CAD build for the part. Positions are in the model's coordinates, mm. Face numbers are marked on the shaded views. A direction names the side the tool comes from. Coordinates: 2 decimals unless noted, no trailing zeros. Loops run counter-clockwise (first coordinate to the right, second up) from the corner with the lowest first, then second, coordinate; pieces in that order, holes last.
1) Saw through at A-A, the plane x = 0. Write the cut outline in (y, z).
2) Saw through at C-C, the plane y = 0. Write the cut outline in (x, z), and give its area (3 significant figures).
3) Pin check, flat tips, straight feed: pin 1 Ø3 at (x, y) = (-18, -100) entering from -Z; pin 2 Ø12 at (x, y) = (2.5, -68.5) entering from -Z; pin 3 Ø4 at (x, y) = (-0.5, -91) entering from -Z; pin 4 Ø12 at (y, z) = (-62.5, -61.5) entering from +X. Stop position of each tip, or through.
4) Saw through at B-B, the plane z = -52.5. Write the cut outline in (x, y).
5) Two-plate mould, pull along Y, no slides. Class the marked faces 5, 6 and 7: +Y half, -Y half, draft (parallel to the pull), parting line (faces both ways), or undercut.
6) Which spindle directions (+Z, -Z, +X, -X, +Y, -Y) get a long thin tool onto all of the face, cutting with end or side? Do the marked faces 1, 2, 3 and 4. Say none if no direction does.
7) Wall check: line 1 along Z through (x, y) = (17.5, 14.5); line 2 along Y through (x, z) = (21.5, -60.5); line 3 along Y through (x, z) = (-19.5, -74.5). Give the ranges that are in metal, low to high.
8) Saw through at D-D, the plane x = -10. Write the cut outline in (y, z), and give its area (3 significant figures).
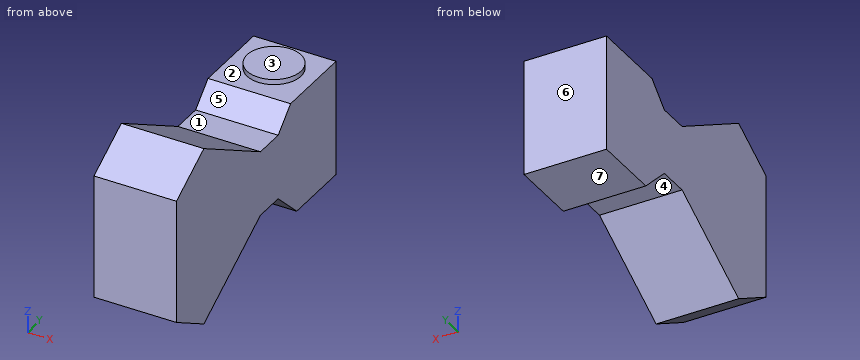
Autodesk Inventor part; units mm, degrees
ref_plane "XZ Plane" through (0, 0, 0) normal (0, 1, 0) x (-1, 0, 0)
sketch "Sketch1" plane through (0, 0, 0) normal (1, 0, 0) x (0, 1, 0)
  line L0 (-16, 3.08) -> (16, 3.08)
  line L1 (16, 3.08) -> (16, 0)
  line L2 (16, 0) -> (-16, 0)
  line L3 (-16, 0) -> (-16, 3.08)
  line L4 (-20.328, 3.08) -> (15.75, 3.08) construction
  line L5 (16, 0) -> (-16, 0) construction
  line L6 (-16, 0) -> (-25.6061, 0)
  line L7 (-25.6061, 0) -> (-38.4616, -12.16)
  line L8 (-38.4616, -12.16) -> (-56.7976, -12.16)
  line L9 (-56.7976, -12.16) -> (-115.4254, 21.9603)
  line L10 (-115.4254, 21.9603) -> (-143.8011, 5.4461)
  line L11 (-143.8011, 5.4461) -> (-143.8011, -68.4461)
  line L12 (-143.8011, -68.4461) -> (-115.4254, -84.9603)
  line L13 (-115.4254, -84.9603) -> (-56.7976, -50.84)
  line L14 (-56.7976, -50.84) -> (-38.4616, -50.84)
  line L15 (-38.4616, -50.84) -> (-19.263, -69)
  line L16 (-19.263, -69) -> (21.5, -69)
  line L17 (21.5, -69) -> (21.5, 0)
  line L18 (21.5, 0) -> (16, 0)
  line L19 (-19.5, -69) -> (19.5, -69) construction
  line L20 (-36.9927, -10.7705) -> (-23.8189, 1.6905) construction
  line L21 (-23.8189, -64.6905) -> (-36.9927, -52.2295) construction
  line L22 (-56.7976, -12.16) -> (-40.4836, -12.16) construction
  line L23 (-40.4836, -50.84) -> (-56.7976, -50.84) construction
  line L24 (-133.6344, 11.4742) -> (-125.5921, 15.9321) construction
  line L25 (-125.5921, -78.9321) -> (-133.6344, -74.4742) construction
  point P0 (0, 0)
  point P1 (0, 0)
  point P2 (21.5, -10)
  point P3 (-129.6132, 13.7032)
  point P4 (-129.6132, -76.7032)
  point P5 (16, 0)
  point P6 (16, 0)
extrude "Extrusion3" add sketch "Sketch1" along normal mid plane 49 contours L2 L18 L17 L16 L15 L14 L13 L12 L11 L10 L9 L8 L7 L6
sketch "Sketch3" plane through (-24.5, -25.6061, 0) normal (0, 0, 1) x (1, 0, 0)
  circle A0 centre (24.5, 25.6061) radius 16
extrude "Extrusion4" add sketch "Sketch3" along normal up to surface (3.08 mm away)
properties part number "BaseBoundingBox"
Data:
1. outline: (-143.8, -68.45) - (-115.43, -84.96) - (-56.8, -50.84) - (-38.46, -50.84) - (-19.26, -69) - (21.5, -69) - (21.5, 0) - (16, 0) - (16, 3.08) - (-16, 3.08) - (-16, 0) - (-25.61, 0) - (-38.46, -12.16) - (-56.8, -12.16) - (-115.43, 21.96) - (-143.8, 5.45) - close
2. outline: (-24.5, -69) - (24.5, -69) - (24.5, 0) - (16, 0) - (16, 3.08) - (-16, 3.08) - (-16, 0) - (-24.5, 0) - close
2. area: 3,480 mm2
3. pin 1: stops at z = -76.86
3. pin 2: stops at z = -61.14
3. pin 3: stops at z = -71.91
3. pin 4: passes through
4. outline: (-24.5, -143.8) - (24.5, -143.8) - (24.5, -59.65) - (-24.5, -59.65) - close; (-24.5, -36.71) - (24.5, -36.71) - (24.5, 21.5) - (-24.5, 21.5) - close
5. face 5: undercut
5. face 6: +Y half
5. face 7: draft
6. face 1: +Z, +X, -X
6. face 2: +Z
6. face 3: +Z, +X, -X, +Y
6. face 4: -Z, +X, -X
7. line 1: z = -69 to 0
7. line 2: y = -143.8 to -73.4, -28.25 to 21.5
7. line 3: y = -133.4 to -97.45
8. outline: (-143.8, -68.45) - (-115.43, -84.96) - (-56.8, -50.84) - (-38.46, -50.84) - (-19.26, -69) - (21.5, -69) - (21.5, 0) - (12.49, 0) - (12.49, 3.08) - (-12.49, 3.08) - (-12.49, 0) - (-25.61, 0) - (-38.46, -12.16) - (-56.8, -12.16) - (-115.43, 21.96) - (-143.8, 5.45) - close
8. area: 11,500 mm2
